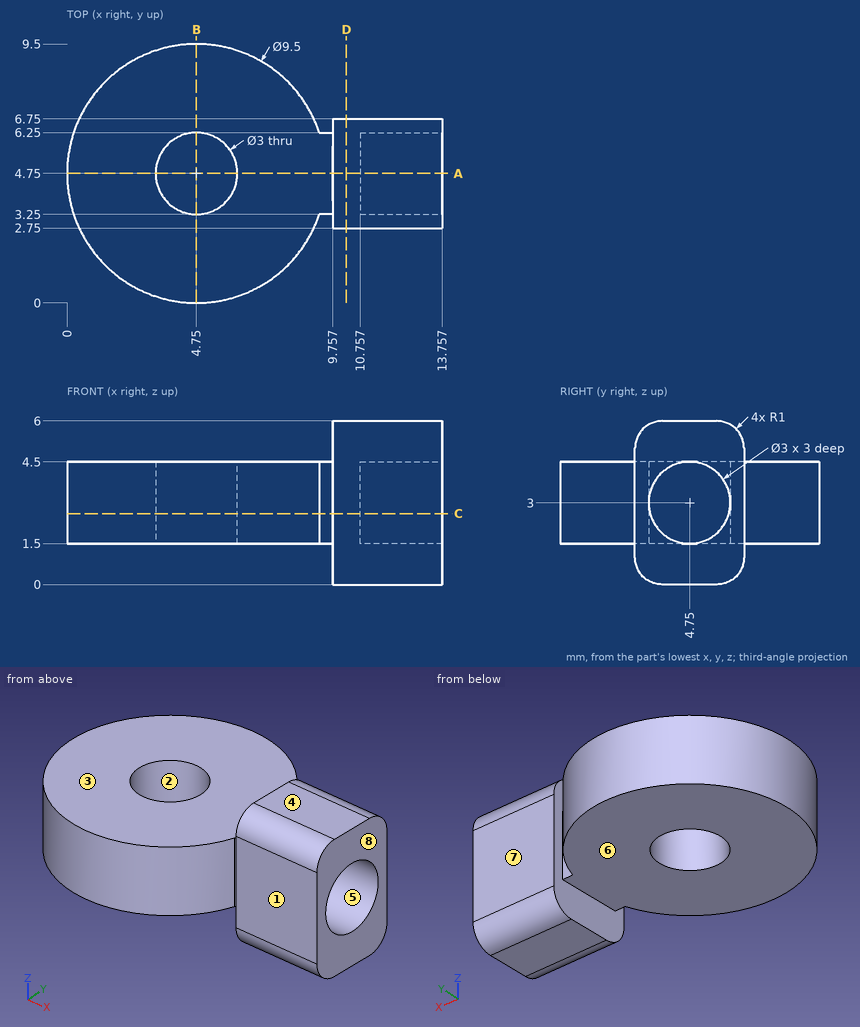
For this review, use the dimensioned drawing (mm, ordinates from the lowest corner) and the shaded views. A direction names the side the tool comes from. Give positions to 0.01 mm unless a question says otherwise; leave off trailing zeros. Order: outer loops, then holes, each group sorted by start corner. A loop starts at its lowest first (then second) coordinate and runs counter-clockwise, first axis right, second up. Notation, with made-up numbers: (3, 61.5) - (30, 61.5) arc R22 ccw to (30, 91.5) - close; hole circle Ø2 at (7.25, 67). An arc over 180 degrees is marked (long way). Use a Markdown table: item, result. Add a question column.
(1) Add section A-A on y = 4.75. Give the boundary of the cut face in (x, z), then the cut area to 3 significant figures.
(2) Add section D-D on x = 10.25. Give the boundary of the cut face in (y, z).
(3) Add section C-C on z = 2.6. Give the boundary of the cut face in (x, y).
(4) Clearance check with flat-ended pins moving along their axes: P1, Ø2, axis at x = 4, y = 8.5, coming from the -Z side; P2, Ø1.5, axis at x = 4, y = 3.5, coming from the +Z side; P3, Ø1.2, axis at y = 5.5, z = 1.5, coming from the -X side. State where each tip first meets the part, or that it passes through.
(5) Machinability: for the marked faces 4, 5, 6, 7 and 8, which of the approach directions +Z, -Z, +X, -X, +Y, -Y give a long, thin tool a straight path to every point of the face, cutting with its end or side? Answer none if there is none.
(6) Mouldability with a two-part tool opening along Y and no side actions: class the marked faces 1, 2 and 3 as +Y half, -Y half, draft (parallel to the pull), parting line (faces both ways), or undercut.
(7) Wall thickness on probe 1 along Y at (x, z) = (4.75, 3.3); probe 2 along Y at (x, z) = (13, 3); probe 3 along Y at (x, z) = (10.75, 1.2): over which ranges is each line inside the solid? List them lowest first. Write a range as [from, to].
(8) Add section B-B on x = 4.75. Give the boundary of the cut face in (y, z), then the cut area to 3 significant figures.
Report:
| question | item | result |
|---|---|---|
| 1 | outline | (0, 1.5) - (3.25, 1.5) - (3.25, 4.5) - (0, 4.5) - close; (6.25, 1.5) - (9.76, 1.5) - (9.76, 0) - (13.76, 0) - (13.76, 1.5) - (10.76, 1.5) - (10.76, 4.5) - (13.76, 4.5) - (13.76, 6) - (9.76, 6) - (9.76, 4.5) - (6.25, 4.5) - close |
| 1 | area | 35.3 mm² |
| 2 | outline | (2.75, 1) arc R1 ccw to (3.75, 0) - (5.75, 0) arc R1 ccw to (6.75, 1) - (6.75, 5) arc R1 ccw to (5.75, 6) - (3.75, 6) arc R1 ccw to (2.75, 5) - close |
| 3 | outline | (9.26, 3.25) - (9.76, 3.25) - (9.76, 2.75) - (13.76, 2.75) - (13.76, 3.3) - (10.76, 3.3) - (10.76, 6.2) - (13.76, 6.2) - (13.76, 6.75) - (9.76, 6.75) - (9.76, 6.25) - (9.26, 6.25) arc R4.75 ccw (long way) to start; hole circle Ø3 at (4.75, 4.75) |
| 4 | P1 | stops at z = 1.5 |
| 4 | P2 | stops at z = 4.5 |
| 4 | P3 | stops at x = 0 |
| 5 | face 4 | +Z, +X, -X, +Y, -Y |
| 5 | face 5 | +X |
| 5 | face 6 | -Z, -X, +Y, -Y |
| 5 | face 7 | +Z, -Z, +X, +Y |
| 5 | face 8 | +Z, -Z, +X, +Y, -Y |
| 6 | face 1 | -Y half |
| 6 | face 2 | undercut |
| 6 | face 3 | draft |
| 7 | probe 1 | y = [0, 3.25], [6.25, 9.5] |
| 7 | probe 2 | y = [2.75, 3.25], [6.25, 6.75] |
| 7 | probe 3 | y = [2.75, 6.75] |
| 8 | outline | (0, 1.5) - (3.25, 1.5) - (3.25, 4.5) - (0, 4.5) - close; (6.25, 1.5) - (9.5, 1.5) - (9.5, 4.5) - (6.25, 4.5) - close |
| 8 | area | 19.5 mm² |
